from build123d import *

# Parameters (mm, degrees)
SKETCH2_R          = 10.668
EXTRUDE1_DEPTH     = 28.194
EXTRUDE1_DRAFT     = -1.783333333
SKETCH5_OUTSIDE_W  = 100.882
SKETCH5_OUTSIDE_H  = 100.882
SKETCH5_OUTSIDE_R  = 9.362586861
CUT_EXTRUDE1_DEPTH = 33.580879133
CUT_EXTRUDE1_DRAFT = 45
SKETCH8_R          = 17.018
CUT_EXTRUDE4_DEPTH = 26.614719415
SKETCH9_OUTSIDE_W  = 32.068
SKETCH9_OUTSIDE_H  = 32.068
SKETCH9_OUTSIDE_R  = 9.489586861
CUT_EXTRUDE5_DEPTH = 1.360714286
SKETCH10_OUTSIDE_W = 82.558
SKETCH10_OUTSIDE_H = 82.558
SKETCH10_OUTSIDE_R = 9.489586861
CUT_EXTRUDE6_DEPTH = 25.296582495
CUT_EXTRUDE6_DRAFT = -45
EXTRUDE2_DEPTH     = 8.4582
SKETCH7_OUTSIDE_W  = 150.768
SKETCH7_OUTSIDE_H  = 154.058
SKETCH7_OUTSIDE_R  = 11.1125
CUT_EXTRUDE2_DEPTH = 33.934882333
CUT_EXTRUDE2_DRAFT = -60
SKETCH18_OUTSIDE_W = 67.856
SKETCH18_OUTSIDE_H = 71.146
SKETCH18_OUTSIDE_R = 11.1125
EXTRUDE3_DEPTH     = 10
EXTRUDE3_DRAFT     = -60
SKETCH11_R         = 8.5725
CUT_EXTRUDE7_DEPTH = 25.615711208
CUT_EXTRUDE7_DRAFT = -1.783333333
SKETCH16_R         = 8.947540861
CUT_EXTRUDE9_DEPTH = 6.35
CUT_EXTRUDE9_DRAFT = -45
SKETCH17_W         = 17.78
SKETCH17_H         = 8.114228224


with BuildPart() as part:
    # Sketch2 → Extrude1 (with draft: the straight prism first)
    with BuildSketch(Plane(origin=(-14.097, 0, 0), x_dir=(0, 0, -1), z_dir=(1, 0, 0))):
        Circle(SKETCH2_R)
    extrude(amount=EXTRUDE1_DEPTH)
    # Extrude1: the draft: its side faces are tilted about the plane it starts from
    extrude1_sides = [part.faces().sort_by_distance(p)[0] for p in [
        (0, 0, 10.668),
    ]]
    draft(extrude1_sides, Plane(origin=(-14.097, 0, 0), x_dir=(0, 0, -1), z_dir=(1, 0, 0)), EXTRUDE1_DRAFT)


with BuildPart() as cut_extrude1_tool:
    # Sketch5 outside → Cut-Extrude1 (with draft: the straight prism first)
    with BuildSketch(Plane(origin=(-14.097, 0, 0), x_dir=(0, 0, -1), z_dir=(1, 0, 0))):
        Rectangle(SKETCH5_OUTSIDE_W, SKETCH5_OUTSIDE_H)
        Circle(SKETCH5_OUTSIDE_R, mode=Mode.SUBTRACT)
    extrude(amount=CUT_EXTRUDE1_DEPTH)
    # Cut-Extrude1: the draft: its side faces are tilted about the plane it starts from
    cut_extrude1_sides = [cut_extrude1_tool.faces().sort_by_distance(p)[0] for p in [
        (2.693439567, -50.441, 0),
        (2.693439567, 0, -50.441),
        (2.693439567, 50.441, 0),
        (2.693439567, 0, 50.441),
        (2.693439567, 0, 9.362586861),
    ]]
    draft(cut_extrude1_sides, Plane(origin=(-14.097, 0, 0), x_dir=(0, 0, -1), z_dir=(1, 0, 0)), CUT_EXTRUDE1_DRAFT)


with BuildPart() as part_1:
    add(part.part)

    # Cut-Extrude1: cut by cut_extrude1_tool
    add(cut_extrude1_tool.part, mode=Mode.SUBTRACT)

    # Sketch8 → Cut-Extrude4 (cut, through all)
    with BuildSketch(Plane(origin=(5.6388, 0, 0), x_dir=(0, 0, -1), z_dir=(1, 0, 0))):
        Circle(SKETCH8_R)
    extrude(amount=CUT_EXTRUDE4_DEPTH, mode=Mode.SUBTRACT)

    # Sketch9 outside → Cut-Extrude5 (cut)
    with BuildSketch(Plane(origin=(5.6388, 0, 0), x_dir=(0, 0, -1), z_dir=(1, 0, 0))):
        Rectangle(SKETCH9_OUTSIDE_W, SKETCH9_OUTSIDE_H)
        Circle(SKETCH9_OUTSIDE_R, mode=Mode.SUBTRACT)
    extrude(amount=-CUT_EXTRUDE5_DEPTH, mode=Mode.SUBTRACT)


with BuildPart() as cut_extrude6_tool:
    # Sketch10 outside → Cut-Extrude6 (with draft: the straight prism first)
    with BuildSketch(Plane(origin=(4.278085714, 0, 0), x_dir=(0, 0, -1), z_dir=(1, 0, 0))):
        Rectangle(SKETCH10_OUTSIDE_W, SKETCH10_OUTSIDE_H)
        Circle(SKETCH10_OUTSIDE_R, mode=Mode.SUBTRACT)
    extrude(amount=-CUT_EXTRUDE6_DEPTH)
    # Cut-Extrude6: the draft: its side faces are tilted about the plane it starts from
    cut_extrude6_sides = [cut_extrude6_tool.faces().sort_by_distance(p)[0] for p in [
        (-8.370205533, -41.279, 0),
        (-8.370205533, 0, -41.279),
        (-8.370205533, 41.279, 0),
        (-8.370205533, 0, 41.279),
        (-8.370205533, 0, 9.489586861),
    ]]
    draft(cut_extrude6_sides, Plane(origin=(4.278085714, 0, 0), x_dir=(0, 0, -1), z_dir=(1, 0, 0)), CUT_EXTRUDE6_DRAFT)


with BuildPart() as part_2:
    add(part_1.part)

    # Cut-Extrude6: cut by cut_extrude6_tool
    add(cut_extrude6_tool.part, mode=Mode.SUBTRACT)

    # Sketch6 → Extrude2 (add)
    with BuildSketch(Plane(origin=(14.097, 0, 0), x_dir=(0, 0, -1), z_dir=(1, 0, 0))):
        Polygon((0, 12.831609733), (-11.1125, 6.415804866), (-11.1125, -6.415804866), (0, -12.831609733), (11.1125, -6.415804866), (11.1125, 6.415804866), align=None)
    extrude(amount=-EXTRUDE2_DEPTH)


with BuildPart() as cut_extrude2_tool:
    # Sketch7 outside → Cut-Extrude2 (with draft: the straight prism first)
    with BuildSketch(Plane(origin=(14.097, 0, 0), x_dir=(0, 0, -1), z_dir=(1, 0, 0))):
        Rectangle(SKETCH7_OUTSIDE_W, SKETCH7_OUTSIDE_H)
        Circle(SKETCH7_OUTSIDE_R, mode=Mode.SUBTRACT)
    extrude(amount=-CUT_EXTRUDE2_DEPTH)
    # Cut-Extrude2: the draft: its side faces are tilted about the plane it starts from
    cut_extrude2_sides = [cut_extrude2_tool.faces().sort_by_distance(p)[0] for p in [
        (-2.870441167, -77.029, 0),
        (-2.870441167, 0, -75.384),
        (-2.870441167, 77.029, 0),
        (-2.870441167, 0, 75.384),
        (-2.870441167, 0, 11.1125),
    ]]
    draft(cut_extrude2_sides, Plane(origin=(14.097, 0, 0), x_dir=(0, 0, -1), z_dir=(1, 0, 0)), CUT_EXTRUDE2_DRAFT)


with BuildPart() as part_3:
    add(part_2.part)

    # Cut-Extrude2: cut by cut_extrude2_tool
    add(cut_extrude2_tool.part, mode=Mode.SUBTRACT)


with BuildPart() as extrude3_tool:
    # Sketch18 outside → Extrude3 (with draft: the straight prism first)
    with BuildSketch(Plane.ZY.offset(-5.6388)):
        Rectangle(SKETCH18_OUTSIDE_W, SKETCH18_OUTSIDE_H)
        Circle(SKETCH18_OUTSIDE_R, mode=Mode.SUBTRACT)
    extrude(amount=-EXTRUDE3_DEPTH)
    # Extrude3: the draft: its side faces are tilted about the plane it starts from
    extrude3_sides = [extrude3_tool.faces().sort_by_distance(p)[0] for p in [
        (10.6388, -35.573, 0),
        (10.6388, 0, 33.928),
        (10.6388, 35.573, 0),
        (10.6388, 0, -33.928),
        (10.6388, 0, -11.1125),
    ]]
    draft(extrude3_sides, Plane.ZY.offset(-5.6388), EXTRUDE3_DRAFT)


with BuildPart() as part_4:
    add(part_3.part)

    # Extrude3: cut by extrude3_tool
    add(extrude3_tool.part, mode=Mode.SUBTRACT)


with BuildPart() as cut_extrude7_tool:
    # Sketch11 → Cut-Extrude7 (with draft: the straight prism first)
    with BuildSketch(Plane(origin=(3.683, 0, 0), x_dir=(0, 0, -1), z_dir=(1, 0, 0))):
        Circle(SKETCH11_R)
    extrude(amount=CUT_EXTRUDE7_DEPTH)
    # Cut-Extrude7: the draft: its side faces are tilted about the plane it starts from
    cut_extrude7_sides = [cut_extrude7_tool.faces().sort_by_distance(p)[0] for p in [
        (16.490855604, 0, 8.5725),
    ]]
    draft(cut_extrude7_sides, Plane(origin=(3.683, 0, 0), x_dir=(0, 0, -1), z_dir=(1, 0, 0)), CUT_EXTRUDE7_DRAFT)


with BuildPart() as part_5:
    add(part_4.part)

    # Cut-Extrude7: cut by cut_extrude7_tool
    add(cut_extrude7_tool.part, mode=Mode.SUBTRACT)


with BuildPart() as cut_extrude9_tool:
    # Sketch16 → Cut-Extrude9 (with draft: the straight prism first)
    with BuildSketch(Plane(origin=(14.097, 0, 0), x_dir=(0, 0, -1), z_dir=(1, 0, 0))):
        Circle(SKETCH16_R)
    extrude(amount=-CUT_EXTRUDE9_DEPTH)
    # Cut-Extrude9: the draft: its side faces are tilted about the plane it starts from
    cut_extrude9_sides = [cut_extrude9_tool.faces().sort_by_distance(p)[0] for p in [
        (10.922, 0, 8.947540861),
    ]]
    draft(cut_extrude9_sides, Plane(origin=(14.097, 0, 0), x_dir=(0, 0, -1), z_dir=(1, 0, 0)), CUT_EXTRUDE9_DRAFT)


with BuildPart() as part_6:
    add(part_5.part)

    # Cut-Extrude9: cut by cut_extrude9_tool
    add(cut_extrude9_tool.part, mode=Mode.SUBTRACT)

    # Sketch17 → Cut-Revolve1 (revolve, cut)
    with BuildSketch(Plane.XY, mode=Mode.PRIVATE) as cut_revolve1_sk:
        with Locations((-5.207, 4.057114112)):
            Rectangle(SKETCH17_W, SKETCH17_H)
    revolve(cut_revolve1_sk.sketch.rotate(Axis((-14.097, 0, 0), (1, 0, 0)), 90), axis=Axis((-14.097, 0, 0), (1, 0, 0)), mode=Mode.SUBTRACT)


solid = part_6.part
Build history of the part. All positions in model axes, mm. A direction names the side the tool comes from. Coordinates: 2 decimals unless noted, no trailing zeros. Order: outer loops, then holes, each group sorted by start corner. A loop starts at its lowest first (then second) coordinate and runs counter-clockwise, first axis right, second up. Notation, with made-up numbers: M 73,-20 L 123,-20 A3 cw 123,-15 Z; hole C 25,40 d6. An arc over 180 degrees is marked long. One line per question, with ' | ' between items. Start each with the question number.
Q1. Flat gauge pins, fed straight in: pin 1 Ø4 at (x, y) = (1, 7) entering from -Z; pin 2 Ø4 at (x, y) = (8.5, -0.5) entering from +Z; pin 3 Ø12 at (x, y) = (9.5, 4) entering from -Z; pin 4 Ø8.5 at (y, z) = (-3, 4.5) entering from +X. Where does each tip first touch, or does it go through?
Q2. Saw through at A-A (x = 10.75). List the corners of the cut face in (y, z).
Q3. Probe L1, parallel to Y at x = 0, z = 0; L2, parallel to X at y = 4.5, z = 7; L3, parallel to Y at x = 4, z = 6.5. List the from-to ranges inside material, lowest first. Write a range as from..to.
Q4. Two-plate mould, pull along Z, no slides. Class faces 1 (the face through (5.875, -5.737, -9.993)), 2 (the face through (-14.097, 8, 3)), 3 (the face through (8.79, 2.62, -8.33)), 4 (the face through (5.875, -5.786, 9.965)): +Z half, -Z half, draft (parallel to the pull), parting line (faces both ways), or undercut.
Q5. Saw through at B-B (x = -6.5). List the corners of the cut face in (y, z).
Q6. 3-axis set-ups, long thin cutter, end or side, ignore diameter. For faces 5 (the face through (10, 0, -11.112)), 6 (the face through (10, 0, 11.112)), 7 (the face through (5.875, 11.522, 0.028)), 8 (the face through (9.93, -9.67, -5.48)): which of +Z, -Z, +X, -X, +Y, -Y reach the whole face in a straight line?
Check values:
1) pin 1: stops at z = -9.96 | pin 2: stops at z = 11.11 | pin 3: stops at z = -11.11 | pin 4: stops at x = 14.1
2) outline: M -12.83,0 L -6.42,-11.11 L 6.42,-11.11 L 12.83,0 L 6.42,11.11 L -6.42,11.11 Z; hole C 0,0 d17.59
3) L1: y = -11.11..-8.11, 8.11..11.11 | L2: x = -14.1..3.68 | L3: y = -7.29..-5.6, 5.6..7.29
4) face 1: -Z half | face 2: draft | face 3: undercut | face 4: +Z half
5) outline: C 0,0 d21.81; hole C 0,0 d16.23
6) face 5: -Z, +X, +Y, -Y | face 6: +Z, +X, +Y, -Y | face 7: +Y | face 8: -Z, +X, -Y
